```python
from build123d import *

# Parameters (mm, degrees)
F1_DEPTH = 114.3
F3_W     = 95.25
F3_H     = 45.085
F4_DEPTH = 3.175
F6_D     = 27.432
F6_DEPTH = 3.175
F7_DEPTH = 3.175
F8_W     = 95.25
F8_H     = 25.4
F9_DEPTH = 45.086


with BuildPart() as f1:
    # F0 (on Front) → F1 (new body)
    with BuildSketch(Plane.XZ):
        Polygon((-38.070478, -17.257856), (-34.895478, -17.257856), (-34.895478, 24.652144), (54.004522, 24.652144), (54.004522, -17.257856), (57.179522, -17.257856), (57.179522, 27.827144), (-38.070478, 27.827144), align=None)
    extrude(amount=F1_DEPTH)

    # F3 (on face) + F0 (on Front) → F4 (join)
    with BuildSketch(Plane.XZ.offset(114.3)):
        with Locations((9.554522, 5.284644)):
            Rectangle(F3_W, F3_H)
    with BuildSketch(Plane.XZ):
        Polygon((-38.070478, -17.257856), (-34.895478, -17.257856), (-34.895478, 24.652144), (54.004522, 24.652144), (54.004522, -17.257856), (57.179522, -17.257856), (57.179522, 27.827144), (-38.070478, 27.827144), align=None)
        with BuildLine():
            Line((-34.895478, 24.652144), (-34.895478, -17.257856))
            Line((-34.895478, -17.257856), (-32.609478, -17.257856))
            Line((-32.609478, -17.257856), (-32.609478, 9.669455))
            ThreePointArc((-32.609478, 9.669455), (-18.893478, 21.604144), (-5.177478, 9.669455))
            Line((-5.177478, 9.669455), (-5.177478, -17.257856))
            Line((-5.177478, -17.257856), (54.004522, -17.257856))
            Line((54.004522, -17.257856), (54.004522, 24.652144))
            Line((54.004522, 24.652144), (-34.895478, 24.652144))
        make_face()
        with BuildLine():
            Line((-32.609478, 9.669455), (-32.609478, -17.257856))
            Line((-32.609478, -17.257856), (-5.177478, -17.257856))
            Line((-5.177478, -17.257856), (-5.177478, 9.669455))
            ThreePointArc((-5.177478, 9.669455), (-18.893478, 21.604144), (-32.609478, 9.669455))
        make_face()
    extrude(amount=F4_DEPTH)

    # F6
    with Locations(Plane(origin=(0, 0, 0), x_dir=(1, 0, 0), z_dir=(0, 1, 0))):
        with Locations((-21.159343, 10.779062)):
            Hole(F6_D / 2, depth=F6_DEPTH)

    # F5 (on face) → F7 (cut)
    with BuildSketch(Plane.XZ):
        with BuildLine():
            Line((-34.875343, 10.779062), (-7.443343, 10.779062))
            ThreePointArc((-7.443343, 10.779062), (-21.159343, 24.495062), (-34.875343, 10.779062))
        make_face()
        with BuildLine():
            Line((-7.443343, -18.13873), (-7.443343, 10.779062))
            ThreePointArc((-7.443343, 10.779062), (-21.159343, -2.936938), (-34.875343, 10.779062))
            Line((-34.875343, 10.779062), (-34.875343, -18.13873))
            Line((-34.875343, -18.13873), (-7.443343, -18.13873))
        make_face()
    extrude(amount=F7_DEPTH, mode=Mode.SUBTRACT)

    # F8 (on face) → F9 (cut, through all)
    with BuildSketch(Plane.XY.offset(27.827144)):
        with Locations((9.554522, -12.7)):
            Rectangle(F8_W, F8_H)
    extrude(amount=-F9_DEPTH, mode=Mode.SUBTRACT)


solid = f1.part
```
Can you work these out from the model? Positions are in its coordinate system, mm. A direction names the side the tool comes from. Round coordinates to 2 decimals unless told otherwise and drop trailing zeros. Loops run counter-clockwise (first coordinate to the right, second up) from the corner with the lowest first, then second, coordinate; pieces in that order, holes last. Notation, with made-up numbers: (79.25, 85.5) -> (119.25, 85.5) arc R9 ccw to (119.25, 96.5) -> close; hole circle Ø4 at (79, -19). An arc over 180 degrees is marked (long way). One line per item, written item: value. Start each with the question number.
1. If we section it at A-A, the plane x = -18: Write out the boundary of the cut face in (y, z) (3 decimals).
2. For pin 1 (1 mm diameter, centred on x = -16.5, z = 0, fed in from +Y); pin 2 (5 mm diameter, centred on x = -6, y = -69.5, fed in from -Z), each with a flat end and sliding along its axis, tell me the tip position at first contact or that it passes through.
3. If we mould it in two halves opening along X, with no side actions, what happens to faces 3 (the flat face through (-38.07, -71, 5)), 4 (the flat face through (6, -25.4, 25)), 5 (the flat face through (-34.895, -69, 3))? For each: pulls with the +X half, pulls with the -X half, needs draft (parallel to the pull), parting line crosses it, or undercut.
4. If I drill on probe 1 along X at (y, z) = (-48, -8.5); probe 2 along Z at (x, y) = (51, -53.5); probe 3 along Y at (x, z) = (-16.5, -13) (3 decimals), over which ranges is the centre line in solid material (lowest first)?
5. If we section it at C-C, the plane y = -41.5: Write out the boundary of the cut face in (x, z), then the cut area to 3 significant figures.
6. If we section it at B-B, the plane z = -11: Write out the boundary of the cut face in (x, y) (3 decimals), then the cut area to 3 significant figures.
7. For faces 1 (the flat face through (9, -71, 27.827)), 2 (the flat face through (9, -69, 24.652)), which set-ups out of +Z, -Z, +X, -X, +Y, -Y let a thin tool reach every point of the face, with its end or its side?
Calculated:
1. outline: (-117.475, -17.258) -> (-114.3, -17.258) -> (-114.3, 24.652) -> (-25.4, 24.652) -> (-25.4, 27.827) -> (-117.475, 27.827) -> close
2. pin 1: stops at y = -114.3
2. pin 2: stops at z = 24.65
3. face 3: pulls with the -X half
3. face 4: needs draft
3. face 5: undercut
4. probe 1: x = -38.07 to -34.9, 54 to 57.18
4. probe 2: z = 24.65 to 27.83
4. probe 3: y = -117.475 to -114.3
5. outline: (-38.07, -17.26) -> (-34.9, -17.26) -> (-34.9, 24.65) -> (54, 24.65) -> (54, -17.26) -> (57.18, -17.26) -> (57.18, 27.83) -> (-38.07, 27.83) -> close
5. area: 569 mm²
6. outline: (-38.07, -117.475) -> (57.18, -117.475) -> (57.18, -25.4) -> (54.005, -25.4) -> (54.005, -114.3) -> (-34.895, -114.3) -> (-34.895, -25.4) -> (-38.07, -25.4) -> close
6. area: 867 mm²
7. face 1: +Z, +X, -X, +Y, -Y
7. face 2: -Z, +Y
